Work out the finished part from the listing and answer in its coordinate system (mm). Face numbers are marked on the shaded views. A direction names the side the tool comes from. Give positions to 0.01 mm unless a question says otherwise; leave off trailing zeros. One line per question, with ' | ' between items. Start each with the question number.
1. Which of the six approach directions +Z, -Z, +X, -X, +Y, -Y give full straight-line access (tool end or side, diameter ignored) to the marked faces 1, 2 and 3?
2. Each of these flat-tipped pins is pushed along its axis until it touches: pin 1 (1.7 mm diameter, centred on x = 113.5, z = -7, fed in from +Y); pin 2 (3 mm diameter, centred on x = 180, y = 3, fed in from +Z); pin 3 (1 mm diameter, centred on x = 43.5, y = 5.5, fed in from +Z); pin 4 (2 mm diameter, centred on y = 3, z = 3, fed in from +X). Where does it stop, or does it pass through?
3. Find the intervals of material crossed by line 1 (X direction, y = 2, z = -10.5); line 2 (X direction, y = 15.25, z = -4.5); line 3 (Y direction, x = 79.5, z = -0.25) (3 decimals), in increasing order.
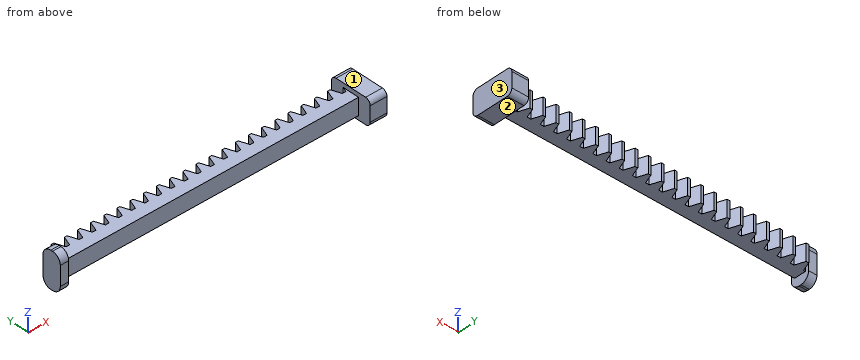
from build123d import *

# Parameters (mm, degrees)
BLANKSKE_W         = 175
BLANKSKE_H         = 12.5
BLANK_DEPTH        = 10
TOOTHCUTSIM_DEPTH  = 176.730617708
TEETHCUTS_COUNT    = 23
TEETHCUTS_PITCH    = 7.853981625
BOSS_EXTRU_1_DEPTH = 5
BOSS_EXTRU_2_DEPTH = 10


with BuildPart() as part:
    # BlankSke → Blank (new body)
    with BuildSketch(Plane.XY):
        with Locations((87.5, 6.25)):
            Rectangle(BLANKSKE_W, BLANKSKE_H)
    extrude(amount=-BLANK_DEPTH)

    # TooCutSkeSim → ToothCutSim (cut, through all)
    with BuildSketch(Plane.XY):
        Polygon((1.087088424, 6.875), (-1.087088424, 6.875), (-3.143665836, 12.5254), (3.143665836, 12.5254), align=None)
    toothcutsim = extrude(amount=-TOOTHCUTSIM_DEPTH, mode=Mode.SUBTRACT)

    # TeethCuts: ToothCutSim ×23
    with Locations(*[(i * TEETHCUTS_PITCH, 0, 0) for i in range(1, TEETHCUTS_COUNT)]):
        add(toothcutsim, mode=Mode.SUBTRACT)

    # Esquisse1 → Boss.-Extru.1 (add)
    with BuildSketch(Plane.ZY):
        with BuildLine():
            Line((-10.736438124, 9.003272752), (0.736438124, 9.003272752))
            ThreePointArc((0.736438124, 9.003272752), (4.27197203, 7.538806658), (5.736438124, 4.003272752))
            Line((5.736438124, 4.003272752), (5.736438124, 2.871727248))
            ThreePointArc((5.736438124, 2.871727248), (4.27197203, -0.663806658), (0.736438124, -2.128272752))
            Line((0.736438124, -2.128272752), (-10.736438124, -2.128272752))
            ThreePointArc((-10.736438124, -2.128272752), (-14.27197203, -0.663806658), (-15.736438124, 2.871727248))
            Line((-15.736438124, 2.871727248), (-15.736438124, 4.003272752))
            ThreePointArc((-15.736438124, 4.003272752), (-14.27197203, 7.538806658), (-10.736438124, 9.003272752))
        make_face()
    extrude(amount=BOSS_EXTRU_1_DEPTH)

    # Esquisse2 → Boss.-Extru.2 (add)
    with BuildSketch(Plane(origin=(175, 0, 0), x_dir=(0, 0, -1), z_dir=(1, 0, 0))):
        with BuildLine():
            Line((9.5, 17.483389911), (0.5, 17.483389911))
            ThreePointArc((0.5, 17.483389911), (-1.621320344, 16.604710254), (-2.5, 14.483389911))
            Line((-2.5, 14.483389911), (-2.5, -4.516610089))
            ThreePointArc((-2.5, -4.516610089), (-1.621320344, -6.637930433), (0.5, -7.516610089))
            Line((0.5, -7.516610089), (9.5, -7.516610089))
            ThreePointArc((9.5, -7.516610089), (11.621320344, -6.637930433), (12.5, -4.516610089))
            Line((12.5, -4.516610089), (12.5, 14.483389911))
            ThreePointArc((12.5, 14.483389911), (11.621320344, 16.604710254), (9.5, 17.483389911))
        make_face()
    extrude(amount=BOSS_EXTRU_2_DEPTH)


solid = part.part
Conclusion:
1) face 1: +Z, +X, +Y, -Y | face 2: -Z, +X, +Y, -Y | face 3: +Z, -Z, +X, +Y, -Y
2) pin 1: y = 12.5 | pin 2: z = 2.5 | pin 3: z = 0 | pin 4: x = 185
3) line 1: -5 to 0, 175 to 185 | line 2: 175 to 185 | line 3: 0 to 6.875
